Geometry: final body of the model. Coordinates: model frame, mm. Face numbers are marked on the shaded views. A direction names the side the tool comes from. Coordinates: 2 decimals unless noted, no trailing zeros. Order: outer loops, then holes, each group sorted by start corner. A loop starts at its lowest first (then second) coordinate and runs counter-clockwise, first axis right, second up. Notation, with made-up numbers: M 74.5,-33 L 128.5,-33 A7 cw 128.5,-25 Z; hole C 73,-18 d8. An arc over 180 degrees is marked long. Use CSV: the item, a comma, the result in double quotes. Start each with the question number.
1. Section query A-A on z = 1.75. Return the cut outline in (x, y).
2. Section query D-D on y = -3.25. Return the cut outline in (x, z), and give its area (3 significant figures).
3. Section query C-C on x = 0. Return the cut outline in (y, z).
4. Set-up query: the marked faces 4, 5, 6 and 7. Return all of +Z, -Z, +X, -X, +Y, -Y with unobstructed straight access to the full face (end or side cutting, diameter ignored); none if empty.
5. Pull-direction query (Z, two-part tool) for the marked faces 1, 2 and 3; classes: pulls with the +Z half, pulls with the -Z half, needs draft (parallel to the pull), parting line crosses it, or undercut.
6. Material intervals for line 1 (Z direction, x = -7.5, y = 4); line 2 (Y direction, x = 0, z = -0.05); line 3 (Y direction, x = 0, z = 0.25), sorted ascending.
7. Section query B-B on y = 1. Return the cut outline in (x, z).
8. First-contact query: P1, Ø1.5, axis at y = 3, z = 2, coming from the +X side; P2, Ø1.5, axis at x = 7, y = -6.5, coming from the -Z side. Flat tips, straight axial feed; report the tip coordinate or a pass-through.
from build123d import *

# Parameters (mm, degrees)
EXTRUDE_1_DEPTH     = 2
SKETCH_2_R          = 9
EXTRUDE_2_DEPTH     = 1
EXTRUDE_START       = 1
SKETCH_3_R          = 9
EXTRUDE_3_DEPTH     = 1
SKETCH_4_R          = 1.5
CUT_EXTRUDE_1_DEPTH = 14.341664064


with BuildPart() as part:
    # Эскиз1 → Бобышка-Вытянуть1 (new body)
    with BuildSketch(Plane.XY):
        Polygon((8.144765867, 0.441612145), (7.35578483, 3.52486338), (5.446952233, 6.071486118), (2.708870535, 7.693780133), (-0.441612145, 8.144765867), (-3.52486338, 7.35578483), (-6.071486118, 5.446952233), (-7.693780133, 2.708870535), (-8.144765867, -0.441612145), (-7.35578483, -3.52486338), (-5.446952233, -6.071486118), (-2.708870535, -7.693780133), (0.441612145, -8.144765867), (3.52486338, -7.35578483), (6.071486118, -5.446952233), (7.693780133, -2.708870535), align=None)
    extrude(amount=EXTRUDE_1_DEPTH)

    # Эскиз2 → Бобышка-Вытянуть2 (add)
    with BuildSketch(Plane(origin=(0, 0, 0), x_dir=(-1, 0, 0), z_dir=(0, 0, -1))):
        Circle(SKETCH_2_R)
    extrude(amount=EXTRUDE_2_DEPTH)

    # Эскиз3 → Бобышка-Вытянуть3 (add)
    with BuildSketch(Plane.XY.offset(2).offset(EXTRUDE_START)):
        with Locations(Location((0, 0, 0), (0, 0, 180))):
            Circle(SKETCH_3_R)
    extrude(amount=-EXTRUDE_3_DEPTH)

    # Эскиз4 → Вырез-Вытянуть1 (cut, through all)
    with BuildSketch(Plane.XY.offset(3)):
        Circle(SKETCH_4_R)
    extrude(amount=-CUT_EXTRUDE_1_DEPTH, mode=Mode.SUBTRACT)


solid = part.part
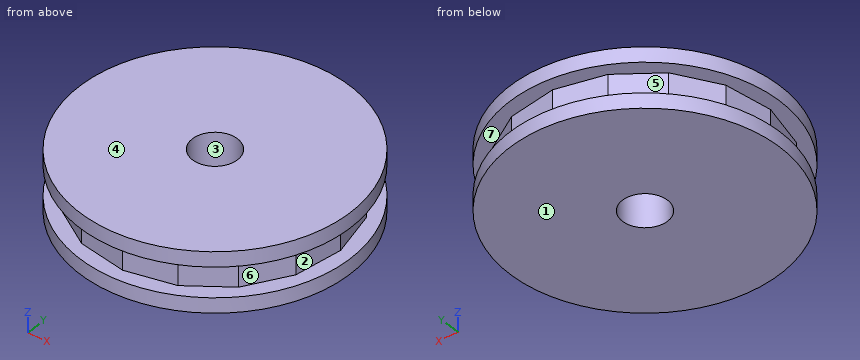
Results list:
1,outline,"M -8.14,-0.44 L -7.36,-3.52 L -5.45,-6.07 L -2.71,-7.69 L 0.44,-8.14 L 3.52,-7.36 L 6.07,-5.45 L 7.69,-2.71 L 8.14,0.44 L 7.36,3.52 L 5.45,6.07 L 2.71,7.69 L -0.44,8.14 L -3.52,7.36 L -6.07,5.45 L -7.69,2.71 Z; hole C 0,0 d3"
2,outline,"M -8.39,-1 L 8.39,-1 L 8.39,0 L 7.37,0 L 7.37,2 L 8.39,2 L 8.39,3 L -8.39,3 L -8.39,2 L -7.43,2 L -7.43,0 L -8.39,0 Z"
2,area,"63.2 mm²"
3,outline,"M -9,-1 L -1.5,-1 L -1.5,3 L -9,3 L -9,2 L -8.08,2 L -8.08,0 L -9,0 Z; M 1.5,-1 L 9,-1 L 9,0 L 8.08,0 L 8.08,2 L 9,2 L 9,3 L 1.5,3 Z"
4,face 4,"+Z, +X, -X, +Y, -Y"
4,face 5,"-X, +Y"
4,face 6,"+X, -Y"
4,face 7,"none"
5,face 1,"pulls with the -Z half"
5,face 2,"undercut"
5,face 3,"needs draft"
6,line 1,"z = -1 to 0, 2 to 3"
6,line 2,"y = -9 to -1.5, 1.5 to 9"
6,line 3,"y = -8.08 to -1.5, 1.5 to 8.08"
7,outline,"M -8.94,-1 L -1.12,-1 L -1.12,3 L -8.94,3 L -8.94,2 L -7.94,2 L -7.94,0 L -8.94,0 Z; M 1.12,-1 L 8.94,-1 L 8.94,0 L 8,0 L 8,2 L 8.94,2 L 8.94,3 L 1.12,3 Z"
8,P1,"stops at x = 8.71"
8,P2,"stops at z = -1"
